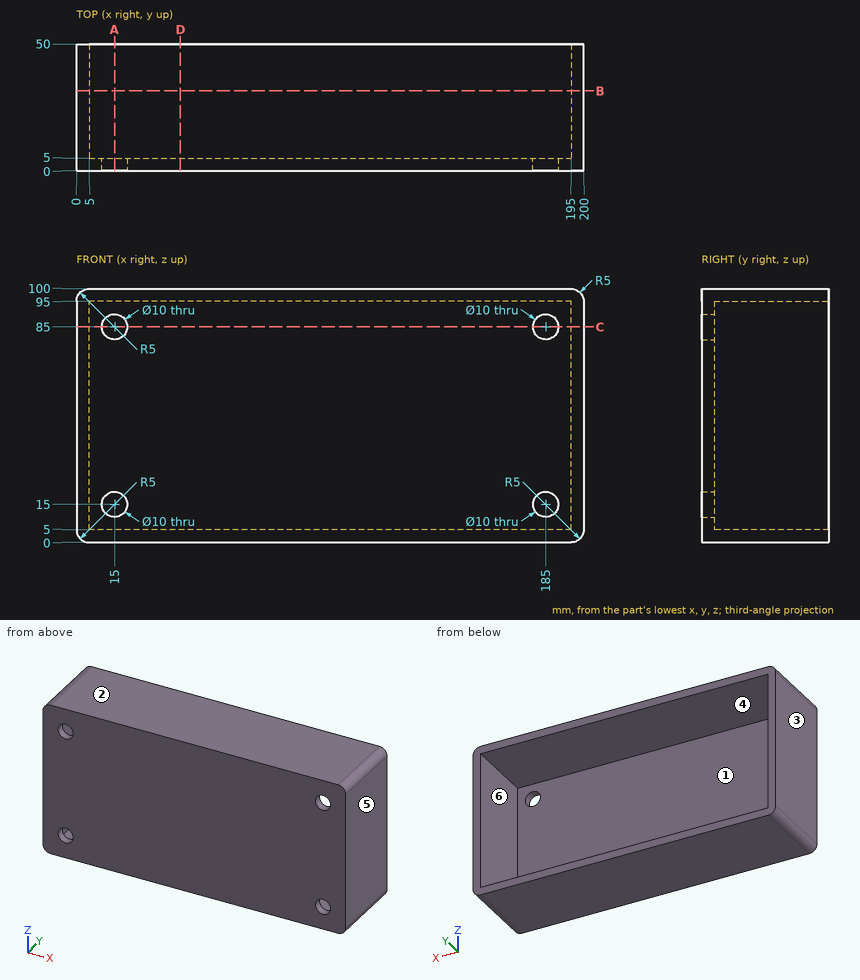
Input: dimensioned drawing with shaded views. Units: mm. Origin: part minimum x, y, z. A direction names the side the tool comes from. Coordinates: 2 decimals unless noted, no trailing zeros. Loops run counter-clockwise (first coordinate to the right, second up) from the corner with the lowest first, then second, coordinate; pieces in that order, holes last. Notation, with made-up numbers: M 14.5,-11 L 62.5,-11 A17 cw 62.5,4 Z; hole C 8,24 d7. An arc over 180 degrees is marked long. One line per item, written item: value. Start each with the question number.
1) Draft query along X for the marked faces 3, 4, 5 and 6. Return one class per face: released by +X, released by -X, zero draft, split by the parting line, or undercut.
2) Cut plane C-C (z = 85). Return loops of the section in (x, y), then the cut area to 3 significant figures.
3) Cut plane A-A (x = 15). Return loops of the section in (y, z), then the cut area to 3 significant figures.
4) Material intervals for L1, parallel to X at y = 4, z = 85; L2, parallel to Z at x = 185, y = 3.6; L3, parallel to Z at x = 101, y = 17, sorted ascending. Write a range as from..to.
5) Cut plane B-B (y = 31.5). Return loops of the section in (x, z), then the cut area to 3 significant figures.
6) Reachability of the marked faces 1 and 2 from +Z, -Z, +X, -X, +Y, -Y: full face, straight path, thin tool, end or side. Return the list, or none.
7) Cut plane D-D (x = 41). Return loops of the section in (y, z).
8) Pin query (flat end, axial travel): P1, Ø16, axis at x = 15, z = 85, coming from the +Y side; P2, Ø9, axis at x = 185, z = 85, coming from the -Y side. Return the tip coordinate at first contact, or that it passes through.
Evaluation:
1. face 3: released by -X
1. face 4: undercut
1. face 5: released by +X
1. face 6: undercut
2. outline: M 0,0 L 10,0 L 10,5 L 5,5 L 5,50 L 0,50 Z; M 20,0 L 180,0 L 180,5 L 20,5 Z; M 190,0 L 200,0 L 200,50 L 195,50 L 195,5 L 190,5 Z
2. area: 1,350 mm^2
3. outline: M 0,0 L 50,0 L 50,5 L 5,5 L 5,10 L 0,10 Z; M 0,20 L 5,20 L 5,80 L 0,80 Z; M 0,90 L 5,90 L 5,95 L 50,95 L 50,100 L 0,100 Z
3. area: 850 mm^2
4. L1: 0..10, 20..180, 190..200
4. L2: 0..10, 20..80, 90..100
4. L3: 0..5, 95..100
5. outline: M 0,5 A5 ccw 5,0 L 195,0 A5 ccw 200,5 L 200,95 A5 ccw 195,100 L 5,100 A5 ccw 0,95 Z; hole M 5,5 L 195,5 L 195,95 L 5,95 Z
5. area: 2,880 mm^2
6. face 1: +Y
6. face 2: +Z, +X, -X, +Y, -Y
7. outline: M 0,0 L 50,0 L 50,5 L 5,5 L 5,95 L 50,95 L 50,100 L 0,100 Z
8. P1: y = 5
8. P2: through
